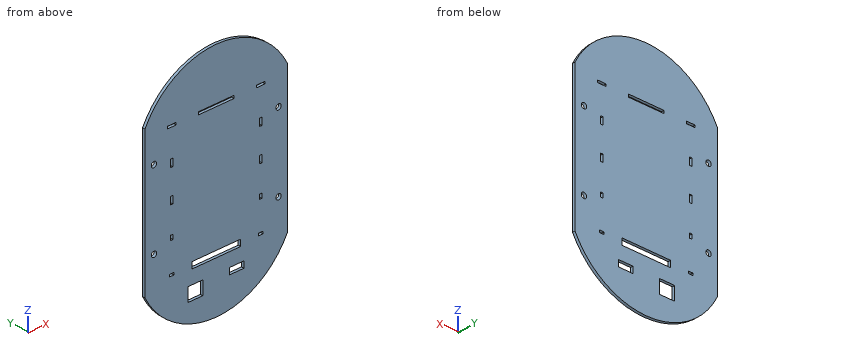
```python
from build123d import *

# Parameters (mm, degrees)
BOSS_EXTRUDE1_DEPTH = 3
SKETCH5_R           = 3
CUT_EXTRUDE2_DEPTH  = 44
SKETCH8_W           = 55
SKETCH8_H           = 7
SKETCH8_W_2         = 2.5
SKETCH8_H_2         = 8
SKETCH8_W_3         = 40
SKETCH8_H_3         = 3
SKETCH8_W_4         = 5
SKETCH8_H_4         = 2.5
SKETCH8_H_5         = 5
SKETCH8_W_5         = 10
CUT_EXTRUDE5_DEPTH  = 31
SKETCH9_W           = 17
SKETCH9_H           = 15
SKETCH9_W_2         = 16
SKETCH9_H_2         = 7
CUT_EXTRUDE6_DEPTH  = 29


with BuildPart() as part:
    # Sketch1 → Boss-Extrude1 (new body)
    with BuildSketch(Plane(origin=(0, 0, 0), x_dir=(1, 0, 0), z_dir=(0, 1, 0))):
        with BuildLine():
            Line((0, 0), (0, 160))
            ThreePointArc((0, 160), (80, 209.178296965), (160, 160))
            Line((160, 160), (160, 0))
            ThreePointArc((160, 0), (80, -49.178296965), (0, 0))
        make_face()
    extrude(amount=BOSS_EXTRUDE1_DEPTH)

    # Sketch5 → Cut-Extrude2 (cut)
    with BuildSketch(Plane(origin=(0, 3, 0), x_dir=(1, 0, 0), z_dir=(0, 1, 0))):
        with Locations(Location((10, 37.5, 0), (0, 0, 270))):
            Circle(SKETCH5_R)
        with Locations(Location((150, 37.5, 0), (0, 0, 270))):
            Circle(SKETCH5_R)
        with Locations(Location((150, 122.5, 0), (0, 0, 270))):
            Circle(SKETCH5_R)
        with Locations(Location((10, 122.5, 0), (0, 0, 270))):
            Circle(SKETCH5_R)
    extrude(amount=-CUT_EXTRUDE2_DEPTH, mode=Mode.SUBTRACT)

    # Sketch8 → Cut-Extrude5 (cut)
    with BuildSketch(Plane(origin=(0, 3, 0), x_dir=(1, 0, 0), z_dir=(0, 1, 0))):
        with Locations((80, 149.5)):
            Rectangle(SKETCH8_W, SKETCH8_H)
        with Locations((30, 43.75)):
            Rectangle(SKETCH8_W_2, SKETCH8_H_2)
        with Locations((80, 8.5)):
            Rectangle(SKETCH8_W_3, SKETCH8_H_3)
        with Locations((30, 149.5)):
            Rectangle(SKETCH8_W_4, SKETCH8_H_4)
        with Locations((130, 149.5)):
            Rectangle(SKETCH8_W_4, SKETCH8_H_4)
        with Locations((130, 114.25)):
            Rectangle(SKETCH8_W_2, SKETCH8_H_5)
        with Locations((30, 114.25)):
            Rectangle(SKETCH8_W_2, SKETCH8_H_5)
        with Locations((30, 79)):
            Rectangle(SKETCH8_W_2, SKETCH8_H_2)
        with Locations((130, 79)):
            Rectangle(SKETCH8_W_2, SKETCH8_H_2)
        with Locations((30, 8.5)):
            Rectangle(SKETCH8_W_5, SKETCH8_H_4)
        with Locations((130, 8.5)):
            Rectangle(SKETCH8_W_5, SKETCH8_H_4)
        with Locations((130, 43.75)):
            Rectangle(SKETCH8_W_2, SKETCH8_H_2)
    extrude(amount=-CUT_EXTRUDE5_DEPTH, mode=Mode.SUBTRACT)

    # Sketch9 → Cut-Extrude6 (cut)
    with BuildSketch(Plane(origin=(0, 3, 0), x_dir=(1, 0, 0), z_dir=(0, 1, 0))):
        with Locations((56.5, 175.5)):
            Rectangle(SKETCH9_W, SKETCH9_H)
        with Locations((103, 171.5)):
            Rectangle(SKETCH9_W_2, SKETCH9_H_2)
    extrude(amount=-CUT_EXTRUDE6_DEPTH, mode=Mode.SUBTRACT)


solid = part.part
```
The model under review builds one solid part; all positions refer to its coordinate system, in mm. Round coordinates to 2 decimals unless told otherwise and drop trailing zeros. Order: outer loops, then holes, each group sorted by start corner. A loop starts at its lowest first (then second) coordinate and runs counter-clockwise, first axis right, second up. Notation, with made-up numbers: (37, 74) -> (76, 74) arc R10 cw to (76, 87) -> close; hole circle Ø5 at (-28.5, -17.75). An arc over 180 degrees is marked (long way). One line per item, written item: value. Start each with the question number.
Q1. Clearance check with flat-ended pins moving along their axes: pin 1 Ø1.5 at (x, y) = (55.5, 1.5) entering from -Z; pin 2 Ø1.5 at (x, y) = (31.5, 2.5) entering from +Z; pin 3 Ø1.5 at (x, y) = (130.5, 2) entering from -Z; pin 4 Ø3.5 at (x, z) = (150, -122.5) entering from +Y. State where each tip first meets the part, or that it passes through.
Q2. Take a section at B-B (x = 10). Write out the cut boundary in (y, z).
Q3. Wall thickness on line 1 (X direction, y = 2.25, z = -37.5); line 2 (Z direction, x = 69.5, y = 0.9); line 3 (Z direction, x = 150, y = 0.75): over which ranges is each line inside the solid? List them lowest first.
Q4. Take a section at A-A (z = -122.5). Write out the cut boundary in (x, y).
Q5. Take a section at D-D (x = 116). Write out the cut boundary in (y, z), and give its area (3 significant figures).
Q6. Take a section at C-C (y = 2.4). Count the separate pieces of the cut face and the enclosed holes in it, and give its area (3 significant figures).
Reported:
1. pin 1: stops at z = -205.98
1. pin 2: stops at z = 35.41
1. pin 3: stops at z = -194.11
1. pin 4: passes through
2. outline: (0, -175.54) -> (3, -175.54) -> (3, -125.5) -> (0, -125.5) -> close; (0, -119.5) -> (3, -119.5) -> (3, -40.5) -> (0, -40.5) -> close; (0, -34.5) -> (3, -34.5) -> (3, 15.54) -> (0, 15.54) -> close
3. line 1: x = 0 to 7, 13 to 147, 153 to 160
3. line 2: z = -208.56 to -153, -146 to -10, -7 to 48.56
3. line 3: z = -175.54 to -125.5, -119.5 to -40.5, -34.5 to 15.54
4. outline: (0, 0) -> (7, 0) -> (7, 3) -> (0, 3) -> close; (13, 0) -> (147, 0) -> (147, 3) -> (13, 3) -> close; (153, 0) -> (160, 0) -> (160, 3) -> (153, 3) -> close
5. outline: (0, -201.63) -> (3, -201.63) -> (3, 41.63) -> (0, 41.63) -> close
5. area: 730 mm2
6. separate pieces: 1
6. enclosed holes: 18
6. area: 35,700 mm2
